Source: three-view drawing plus pictorial views. Frame: mm from the lowest corner of the part. A direction names the side the tool comes from. Coordinates: 2 decimals unless noted, no trailing zeros. Write each loop counter-clockwise with the first axis right and the second up, starting at its lowest first coordinate (ties: lowest second). Pieces come first, ordered by that corner, then holes. Notation, with made-up numbers: (6.5, 57) - (42.5, 57) arc R21 cw to (42.5, 62) - close; hole circle Ø11 at (-1.75, -28.75). An arc over 180 degrees is marked (long way). One line per item, written item: value.
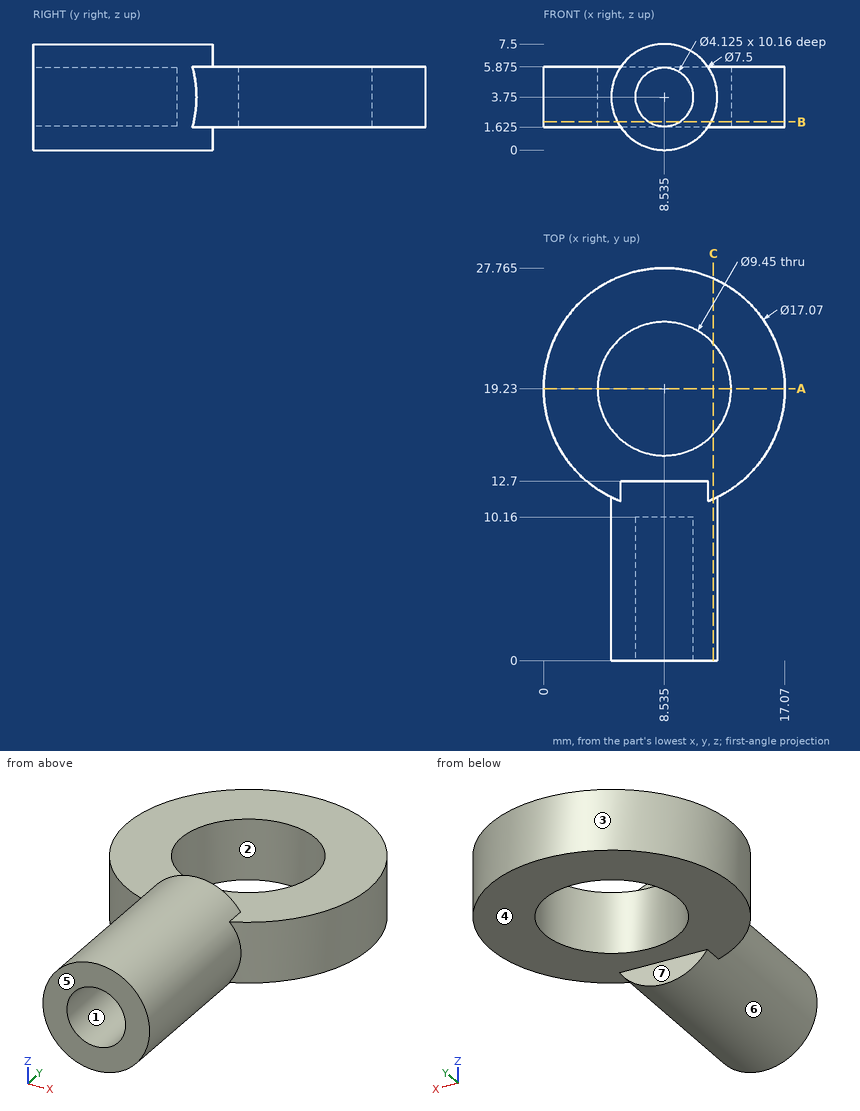
1) Section query B-B on z = 2. Output: boundary loops of the cut face in (x, y) (3 decimals).
Values found:
outline: (5.218, 0) - (7.443, 0) - (7.443, 10.16) - (9.627, 10.16) - (9.627, 0) - (11.852, 0) - (11.852, 11.366) arc R8.535 ccw (long way) to (5.218, 11.366) - close; hole circle Ø9.45 at (8.535, 19.23)
2) Section query C-C on x = 12. Output: boundary loops of the cut face in (y, z) (3 decimals).
Values found:
outline: (0, 2.316) - (11.43, 2.316) - (11.43, 1.625) - (16.018, 1.625) - (16.018, 5.875) - (11.43, 5.875) - (11.43, 5.184) - (0, 5.184) - close; (22.442, 1.625) - (27.03, 1.625) - (27.03, 5.875) - (22.442, 5.875) - close
3) Reachability of the marked faces 5, 6 and 7 from +Z, -Z, +X, -X, +Y, -Y: full face, straight path, thin tool, end or side. Return the list, or none.
Values found:
face 5: +Z, -Z, +X, -X, -Y
face 6: -Y
face 7: -Z, +X, -X, +Y
4) Contact query for flat-ended pins moving along their axis: P1, Ø3, axis at x = 14, y = 18.5, coming from the -Z side (3 decimals); P2, Ø4.5, axis at x = 9, z = 3, coming from the -Y side; P3, Ø6, axis at x = 12.5, y = 6.5, coming from the -Z side; P4, Ø2, axis at x = 5.5, y = 5, coming from the -Z side. Output: stop coordinate, or through.
Values found:
P1: z = 1.625
P2: y = 0
P3: z = 0.13
P4: z = 0.6
5) Draft query along X for the marked faces 1, 2, 3 and 4. Return one class per face: released by +X, released by -X, zero draft, split by the parting line, or undercut.
Values found:
face 1: undercut
face 2: undercut
face 3: split by the parting line
face 4: zero draft
6) Material intervals for line 1 (Y direction, x = 7.75, z = 1); line 2 (Y direction, x = 9.5, z = 3.25); line 3 (X direction, y = 21, z = 1.75), sorted ascending.
Values found:
line 1: 0 to 12.7
line 2: 10.16 to 14.6, 23.86 to 27.71
line 3: 0.19 to 4.15, 12.92 to 16.88
7) Section query A-A on y = 19.23. Output: boundary loops of the cut face in (x, z) (3 decimals).
Values found:
outline: (0, 1.625) - (3.81, 1.625) - (3.81, 5.875) - (0, 5.875) - close; (13.26, 1.625) - (17.07, 1.625) - (17.07, 5.875) - (13.26, 5.875) - close
